Input: part model. Units: mm. Frame: model coordinates. A direction names the side the tool comes from. Round coordinates to 2 decimals unless told otherwise and drop trailing zeros. Order: outer loops, then holes, each group sorted by start corner. A loop starts at its lowest first (then second) coordinate and runs counter-clockwise, first axis right, second up. Notation, with made-up numbers: M 85,76 L 133,76 A15 ccw 133,90 Z; hole C -37,-3 d5. An arc over 180 degrees is marked long. One line per question, with ' | ' between items.
```python
from build123d import *

# Parameters (mm, degrees)
BOSS_EXTRUDE1_DEPTH      = 31.4325
BOSS_EXTRUDE1_DEPTH_BACK = 28.521152
SKETCH1_R                = 22.06625


with BuildPart() as part:
    # Sketch1 → Boss-Extrude1 (new, two sides: drawn at the far end of the back side and taken through both)
    with BuildSketch(Plane.XY.offset(-BOSS_EXTRUDE1_DEPTH_BACK)):
        with BuildLine():
            Line((-112.5601, 40.79875), (-112.5601, -40.79875))
            Line((-112.5601, -40.79875), (-105.64544448, -40.79875))
            Line((-105.64544448, -40.79875), (-78.272997716, -40.79875))
            Line((-78.272997716, -40.79875), (-73.818843223, -40.79875))
            ThreePointArc((-73.818843223, -40.79875), (-72.740595899, -40.954508258), (-71.750509166, -41.40904779))
            ThreePointArc((-71.750509166, -41.40904779), (-71.12778643, -41.911656502), (-70.623783626, -42.533251464))
            Line((-70.623783626, -42.533251464), (-57.043977681, -63.438247804))
            ThreePointArc((-57.043977681, -63.438247804), (-54.978017505, -65.347620641), (-52.251388286, -66.04))
            Line((-52.251388286, -66.04), (-46.145505176, -66.04))
            ThreePointArc((-46.145505176, -66.04), (-43.125397449, -65.176821752), (-41.017587638, -62.848031257))
            Line((-41.017587638, -62.848031257), (-31.215934729, -42.926729162))
            ThreePointArc((-31.215934729, -42.926729162), (-29.810728189, -41.374202165), (-27.797323037, -40.79875))
            Line((-27.797323037, -40.79875), (-17.4625, -40.79875))
            ThreePointArc((-17.4625, -40.79875), (-14.768423164, -41.914673164), (-13.6525, -44.60875))
            Line((-13.6525, -44.60875), (-13.6525, -53.6575))
            ThreePointArc((-13.6525, -53.6575), (-11.048679285, -59.943679285), (-4.7625, -62.5475))
            Line((-4.7625, -62.5475), (4.7625, -62.5475))
            ThreePointArc((4.7625, -62.5475), (11.048679285, -59.943679285), (13.6525, -53.6575))
            Line((13.6525, -53.6575), (13.6525, -44.60875))
            ThreePointArc((13.6525, -44.60875), (14.768423164, -41.914673164), (17.4625, -40.79875))
            Line((17.4625, -40.79875), (27.654758859, -40.79875))
            ThreePointArc((27.654758859, -40.79875), (29.719716377, -41.406867671), (31.125494286, -43.037096222))
            Line((31.125494286, -43.037096222), (40.021517431, -62.682480667))
            ThreePointArc((40.021517431, -62.682480667), (42.130184293, -65.127823493), (45.227620571, -66.04))
            Line((45.227620571, -66.04), (54.568047284, -66.04))
            ThreePointArc((54.568047284, -66.04), (58.173789295, -64.758942889), (60.163026865, -61.49008733))
            Line((60.163026865, -61.49008733), (64.407842813, -41.105642371))
            ThreePointArc((64.407842813, -41.105642371), (65.581423361, -39.0573205), (67.73644034, -38.093569694))
            Line((67.73644034, -38.093569694), (95.251064725, -35.178643905))
            ThreePointArc((95.251064725, -35.178643905), (102.949381832, -31.250135269), (106.045, -23.180784951))
            Line((106.045, -23.180784951), (106.045, 23.328923197))
            ThreePointArc((106.045, 23.328923197), (103.018943576, 31.320276275), (95.45872167, 35.302962082))
            Line((95.45872167, 35.302962082), (51.692807067, 40.707788885))
            ThreePointArc((51.692807067, 40.707788885), (50.954843743, 40.77598825), (50.214085398, 40.79875))
            Line((50.214085398, 40.79875), (-70.371619795, 40.79875))
            Line((-70.371619795, 40.79875), (-78.272997716, 40.79875))
            Line((-78.272997716, 40.79875), (-105.64544448, 40.79875))
            Line((-105.64544448, 40.79875), (-112.5601, 40.79875))
        make_face()
        with Locations(Location((0, 0, 0), (0, 0, 180))):
            Circle(SKETCH1_R, mode=Mode.SUBTRACT)
        with BuildLine():
            Line((51.310190607, -26.854733006), (52.037693166, -26.777660684))
            Line((52.037693166, -26.777660684), (53.233388861, -26.650987532))
            ThreePointArc((53.233388861, -26.650987532), (55.664436368, -25.410405857), (56.642, -22.862189968))
            Line((56.642, -22.862189968), (56.642, 22.960948798))
            ThreePointArc((56.642, 22.960948798), (55.686403235, 25.484533981), (53.298964738, 26.742224235))
            Line((53.298964738, 26.742224235), (51.93932935, 26.910131015))
            Line((51.93932935, 26.910131015), (51.211826791, 26.999973199))
            Line((51.211826791, 26.999973199), (50.876355003, 27.041401943))
            ThreePointArc((50.876355003, 27.041401943), (50.643313953, 27.062938585), (50.409390265, 27.070126506))
            Line((50.409390265, 27.070126506), (43.95784943, 27.070126506))
            Line((43.95784943, 27.070126506), (38.064512232, 27.070126506))
            ThreePointArc((38.064512232, 27.070126506), (34.741474437, 25.123864634), (34.813450689, 21.273496484))
            ThreePointArc((34.813450689, 21.273496484), (40.796592197, -0.419602974), (34.368525909, -21.985050111))
            ThreePointArc((34.368525909, -21.985050111), (34.236008022, -25.867591825), (37.578038056, -27.848128721))
            Line((37.578038056, -27.848128721), (41.732055975, -27.848128721))
            ThreePointArc((41.732055975, -27.848128721), (41.933030203, -27.84282442), (42.133444836, -27.826926285))
            Line((42.133444836, -27.826926285), (43.35576614, -27.69743239))
            Line((43.35576614, -27.69743239), (51.310190607, -26.854733006))
        make_face(mode=Mode.SUBTRACT)
        with BuildLine():
            Line((-49.309702392, 23.01875), (-64.127923903, 23.01875))
            ThreePointArc((-64.127923903, 23.01875), (-66.710199181, 22.685115268), (-69.122880616, 21.706122911))
            ThreePointArc((-69.122880616, 21.706122911), (-72.902157779, 17.981095156), (-74.287923903, 12.85875))
            Line((-74.287923903, 12.85875), (-74.287923903, -12.85875))
            ThreePointArc((-74.287923903, -12.85875), (-72.902157779, -17.981095156), (-69.122880616, -21.706122911))
            ThreePointArc((-69.122880616, -21.706122911), (-66.710199181, -22.685115268), (-64.127923903, -23.01875))
            Line((-64.127923903, -23.01875), (-49.309702392, -23.01875))
            ThreePointArc((-49.309702392, -23.01875), (-41.270013925, -19.07075526), (-39.47848447, -10.295011682))
            ThreePointArc((-39.47848447, -10.295011682), (-40.79875, 0), (-39.47848447, 10.295011682))
            ThreePointArc((-39.47848447, 10.295011682), (-41.270013925, 19.07075526), (-49.309702392, 23.01875))
        make_face(mode=Mode.SUBTRACT)
        with BuildLine():
            Line((71.12, 12.7), (71.12, -12.7))
            ThreePointArc((71.12, -12.7), (71.199051629, -13.96494266), (71.434976365, -15.210201111))
            ThreePointArc((71.434976365, -15.210201111), (82.54494266, -22.780948371), (91.44, -12.7))
            Line((91.44, -12.7), (91.44, 12.7))
            ThreePointArc((91.44, 12.7), (82.54494266, 22.780948371), (71.434976365, 15.210201111))
            ThreePointArc((71.434976365, 15.210201111), (71.199051629, 13.96494266), (71.12, 12.7))
        make_face(mode=Mode.SUBTRACT)
    extrude(amount=BOSS_EXTRUDE1_DEPTH + BOSS_EXTRUDE1_DEPTH_BACK)


solid = part.part
```
Item 1: Line query: line 1 along Y through (x, z) = (0, -5); line 2 along X through (y, z) = (-57.5, 16); line 3 along X through (y, z) = (6, 0.5) (3 decimals). Output: solid intervals per line, ascending. Write a range as from..to.
Report:
line 1: -62.55..-22.07, 22.07..40.8 | line 2: -60.9..-38.39, -12.78..12.78, 37.67..60.99 | line 3: -112.56..-74.288, -40.355..-21.235, 21.235..40.355, 56.642..71.12, 91.44..106.045
Item 2: Mould query, pull axis Y, two halves, no side actions, for faces 4 (the flat face through (44, 27.07, 1)), 5 (the flat face through (106.045, 0, 1)), 6 (the cylindrical face through (14.739, -41.944, 1.036)). Classes: +Y half, -Y half, draft (parallel to the pull), parting line (faces both ways), or undercut.
Report:
face 4: undercut | face 5: draft | face 6: -Y half
Item 3: Section query C-C, the plane x = 25. Return loops of the section in (y, z), plus the area to 3 significant figures.
Report:
outline: M -40.8,-28.52 L 40.8,-28.52 L 40.8,31.43 L -40.8,31.43 Z | area: 4,890 mm²
Item 4: Section query D-D, the plane z = 9.5. Give the number of separate pieces and of enclosed holes in the cut face, plus the area to 3 significant figures.
Report:
separate pieces: 1 | enclosed holes: 4 | area: 14,400 mm²
Item 5: Section query B-B, the plane x = 0. Return loops of the section in (y, z).
Report:
outline: M -62.55,-28.52 L -22.07,-28.52 L -22.07,31.43 L -62.55,31.43 Z; M 22.07,-28.52 L 40.8,-28.52 L 40.8,31.43 L 22.07,31.43 Z
Item 6: Access query for faces 1 (the flat face through (-13.652, -49, 1)), 2 (the flat face through (56.642, 0, 1)), 3 (the flat face through (-93, -40.799, 1)). Directions: +Z, -Z, +X, -X, +Y, -Y. A direction counts if a zero-diameter tool reaches every point of the face in a straight line with its end or side. Return the directions, or none.
Report:
face 1: +Z, -Z, -Y | face 2: +Z, -Z | face 3: +Z, -Z, -X, -Y
Item 7: Section query A-A, the plane y = 0. Return loops of the section in (x, z) (1 decimal), plus the area to 3 significant figures.
Report:
outline: M -112.6,-28.5 L -74.3,-28.5 L -74.3,31.4 L -112.6,31.4 Z; M -40.8,-28.5 L -22.1,-28.5 L -22.1,31.4 L -40.8,31.4 Z; M 22.1,-28.5 L 40.8,-28.5 L 40.8,31.4 L 22.1,31.4 Z; M 56.6,-28.5 L 71.1,-28.5 L 71.1,31.4 L 56.6,31.4 Z; M 91.4,-28.5 L 106,-28.5 L 106,31.4 L 91.4,31.4 Z | area: 6,280 mm²
Item 8: First-contact query: pin 1 (4.5 mm diameter, centred on x = -57.5, z = 4.5, fed in from -Y); pin 2 (3.5 mm diameter, centred on x = 43, z = -8, fed in from -Y); pin 3 (2 mm diameter, centred on y = -32.5, z = 13.5, fed in from +X). Flat tips, straight axial feed; report the tip coordinate or a pass-through.
Report:
pin 1: y = -65.19 | pin 2: y = -66.02 | pin 3: x = 102.72
